CAD build for the part. Positions are in the model's coordinates, mm. Face numbers are marked on the shaded views. A direction names the side the tool comes from. Round coordinates to 2 decimals unless told otherwise and drop trailing zeros. Loops run counter-clockwise (first coordinate to the right, second up) from the corner with the lowest first, then second, coordinate; pieces in that order, holes last. Notation, with made-up numbers: M -17,16 L -3,16 A32 ccw -3,48 Z; hole C 65,-0.5 d6. An arc over 180 degrees is marked long. Use a Markdown table: item, result. Add a question column.
(1) Band-saw the part on C-C, the plane y = -0.5. Write the cut outline in (x, z), and give its area (3 significant figures).
(2) Band-saw the part on A-A, the plane z = 1.5. Write the cut outline in (x, y).
(3) Band-saw the part on B-B, the plane x = 0. Write the cut outline in (y, z), and give its area (3 significant figures).
(4) Band-saw the part on D-D, the plane z = 5.5. Write the cut outline in (x, y), and give its area (3 significant figures).
(5) Two-plate mould, pull along Y, no slides. Class the marked faces 4, 5 and 6: released by +Y, released by -Y, zero draft, split by the parting line, or undercut.
(6) Wall check: L1, parallel to Y at x = 0.05, z = 0.5; L2, parallel to Y at x = -0.1, z = 4.75; L3, parallel to Z at x = -1.55, y = -3.5. Give the ranges that are in metal, low to high.
(7) Which spindle directions (+Z, -Z, +X, -X, +Y, -Y) get a long thin tool onto all of the face, cutting with end or side? Do the marked faces 1, 2 and 3. Say none if no direction does.
(8) Flat gauge pins, fed straight in: P1, Ø1.6, axis at x = 0, y = 0, coming from the +Z side; P2, Ø1.5, axis at y = -0.5, z = 4, coming from the -X side. Where does each tip first touch, or does it go through?
from build123d import *

# Parameters (mm, degrees)
SKETCH_1_R      = 1
EXTRUDE_1_DEPTH = 2
SKETCH_2_R      = 2
EXTRUDE_2_DEPTH = 6
EXTRUDE_START   = 0.9
SKETCH_3_R      = 1
SKETCH_3_R_2    = 2
EXTRUDE_3_DEPTH = 0.9


with BuildPart() as part:
    # Sketch 1 → Extrude 1 (new body)
    with BuildSketch(Plane.XY):
        Circle(SKETCH_1_R)
    extrude(amount=EXTRUDE_1_DEPTH)



with BuildPart() as body_2:
    # Sketch 2 → Extrude 2 (new body)
    with BuildSketch(Plane(origin=(0, 0, 0), x_dir=(-1, 0, 0), z_dir=(0, 0, -1))):
        with Locations((0, -5)):
            Circle(SKETCH_2_R)
    extrude(amount=-EXTRUDE_2_DEPTH)


with BuildPart() as part_1:
    add(part.part)

    add(body_2.part)  # Extrude 3 merges body 2
    # Sketch 3 → Extrude 3 (add)
    with BuildSketch(Plane(origin=(0, 0, 0), x_dir=(-1, 0, 0), z_dir=(0, 0, -1)).offset(EXTRUDE_START)):
        with Locations(Location((0, 0, 0), (0, 0, 11.536959033))):
            Circle(SKETCH_3_R)
        with BuildLine():
            Line((1.959591794, -4.6), (0.979795897, 0.2))
            ThreePointArc((0.979795897, 0.2), (0.994936153, 0.100508962), (1, 0))
            ThreePointArc((1, 0), (-0.100508962, -0.994936153), (-0.979795897, 0.2))
            Line((-0.979795897, 0.2), (-1.959591794, -4.6))
            ThreePointArc((-1.959591794, -4.6), (0, -3), (1.959591794, -4.6))
        make_face()
        with Locations(Location((0, -5, 0), (0, 0, 168.463040967))):
            Circle(SKETCH_3_R_2)
    extrude(amount=-EXTRUDE_3_DEPTH)


solid = part_1.part
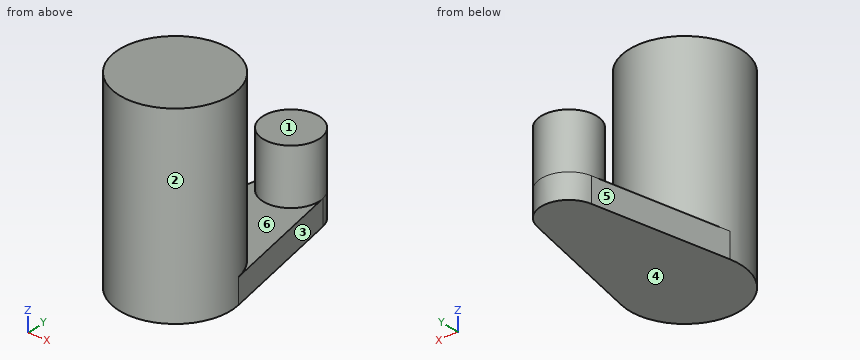
Return value:
| question | item | result |
|---|---|---|
| 1 | outline | M -1.12,-0.9 L 1.12,-0.9 L 1.12,0 L 0.87,0 L 0.87,2 L -0.87,2 L -0.87,0 L -1.12,0 Z |
| 1 | area | 5.48 mm^2 |
| 2 | outline | C 0,-5 d4; C 0,0 d2 |
| 3 | outline | M -7,-0.9 L 1,-0.9 L 1,2 L -1,2 L -1,0 L -3,0 L -3,6 L -7,6 Z |
| 3 | area | 35.2 mm^2 |
| 4 | outline | C 0,-5 d4 |
| 4 | area | 12.6 mm^2 |
| 5 | face 4 | zero draft |
| 5 | face 5 | released by +Y |
| 5 | face 6 | undercut |
| 6 | L1 | -7 to -3, -1 to 1 |
| 6 | L2 | -7 to -3 |
| 6 | L3 | -0.9 to 0 |
| 7 | face 1 | +Z, +X, -X, +Y |
| 7 | face 2 | +Z |
| 7 | face 3 | +Z, -Z, +X, +Y |
| 8 | P1 | z = 2 |
| 8 | P2 | through |
